Model file for the job. Use its own axes, mm. Round coordinates to 2 decimals unless told otherwise and drop trailing zeros. Loops run counter-clockwise (first coordinate to the right, second up) from the corner with the lowest first, then second, coordinate; pieces in that order, holes last. Notation, with made-up numbers: M -4.75,76 L 36.25,76 A16 ccw 36.25,84 Z; hole C 73,-7.5 d8. An arc over 180 degrees is marked long. Use a Markdown table: item, result. Add a question column.
Item 1: Two-plate mould, pull along Z, no slides. Class faces 1 (the flat face through (-5, 5, 2)), 2 (the flat face through (-5, 5, 0)): +Z half, -Z half, draft (parallel to the pull), parting line (faces both ways), or undercut.
Item 2: Wall check: L1, parallel to Z at x = 26, y = -252. Give the ranges that are in metal, low to high. Write a range as from..to.
Item 3: Saw through at B-B on z = -1.3. Write the cut outline in (x, y).
Item 4: Pin check, flat tip, straight feed: P1, Ø3, axis at x = 119.5, y = 122, coming from the -Z side. Stop position of the tip, or through.
Item 5: Saw through at A-A on x = -219.5. Write the cut outline in (y, z), then the cut area to 3 significant figures.
```python
from build123d import *

# Parameters (mm, degrees)
SKETCH1_W           = 720
SKETCH1_H           = 720
BOSS_EXTRUDE1_DEPTH = 2
SKETCH2_R           = 5
BOSS_EXTRUDE2_DEPTH = 2


with BuildPart() as part:
    # Sketch1 → Boss-Extrude1 (new body)
    with BuildSketch(Plane.XY):
        Rectangle(SKETCH1_W, SKETCH1_H)
    extrude(amount=BOSS_EXTRUDE1_DEPTH)

    # Sketch2 → Boss-Extrude2 (add)
    with BuildSketch(Plane(origin=(0, 0, 0), x_dir=(-1, 0, 0), z_dir=(0, 0, -1))):
        with Locations((0, 340)):
            Circle(SKETCH2_R)
        with Locations((-340, 0)):
            Circle(SKETCH2_R)
        with Locations((0, -340)):
            Circle(SKETCH2_R)
        with Locations((340, 0)):
            Circle(SKETCH2_R)
    extrude(amount=BOSS_EXTRUDE2_DEPTH)


solid = part.part
```
Entries:
| question | item | result |
|---|---|---|
| 1 | face 1 | +Z half |
| 1 | face 2 | -Z half |
| 2 | L1 | 0..2 |
| 3 | outline | C -340,0 d10; C 0,-340 d10; C 0,340 d10; C 340,0 d10 |
| 4 | P1 | z = 0 |
| 5 | outline | M -360,0 L 360,0 L 360,2 L -360,2 Z |
| 5 | area | 1,440 mm2 |
